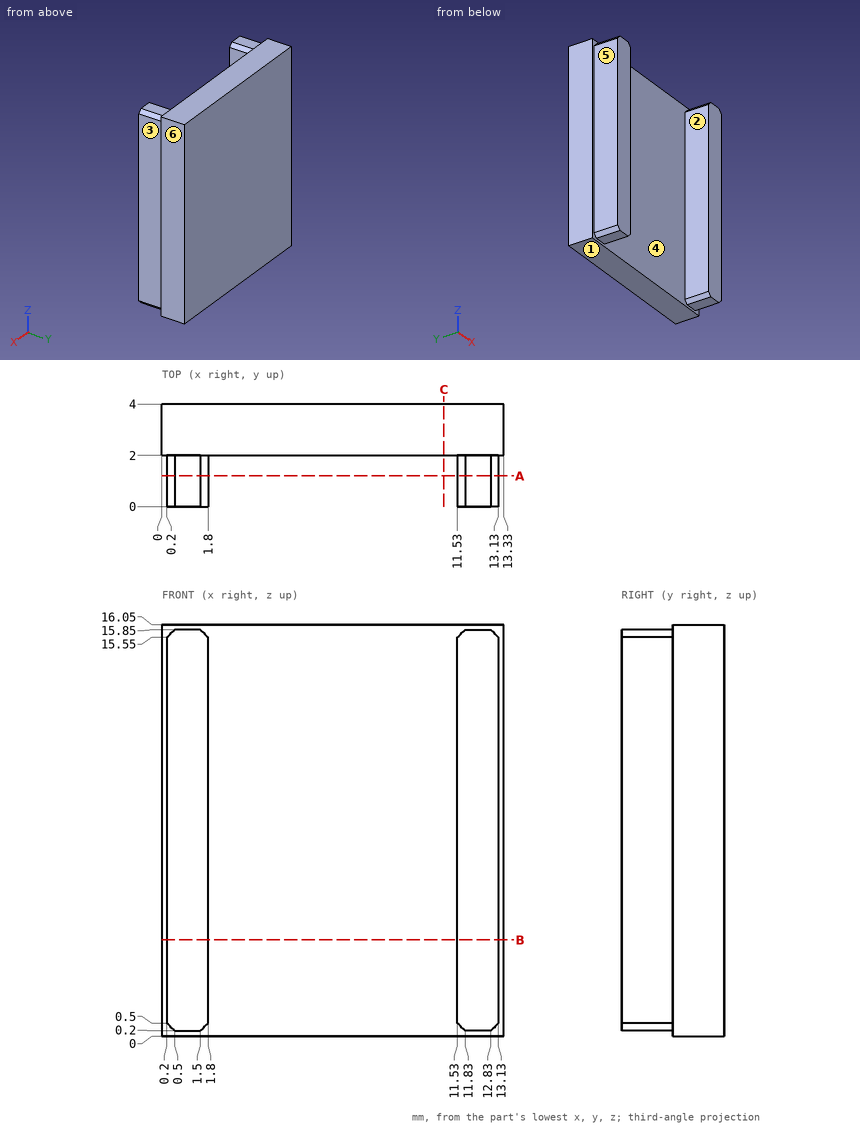
Can you work these out from the drawing? Everything is in mm from the part's minimum corner. A direction names the side the tool comes from. Coordinates: 2 decimals unless noted, no trailing zeros. Loops run counter-clockwise (first coordinate to the right, second up) from the corner with the lowest first, then second, coordinate; pieces in that order, holes last. Notation, with made-up numbers: (46.25, -31.75) - (72.25, -31.75) arc R20 cw to (72.25, -9.75) - close; hole circle Ø9 at (48.25, 11.25). An arc over 180 degrees is marked (long way). Use a Markdown table: item, result.
Item 1: Will these pins go through, and if not, where does the flat tip stop? pin 1 (1.1 mm diameter, centred on x = 12, y = 0.5, fed in from -Z); pin 2 (1.6 mm diameter, centred on y = 1, z = 11.5, fed in from -X).
Numbers:
| item | result |
|---|---|
| pin 1 | stops at z = 0.2 |
| pin 2 | stops at x = 0.2 |
Item 2: I want a section at C-C on x = 11. Please give me the cut outline in (y, z).
Numbers:
| item | result |
|---|---|
| outline | (2, 0) - (4, 0) - (4, 16.05) - (2, 16.05) - close |
Item 3: For the marked faces 1, 2 and 3, which set-ups out of +Z, -Z, +X, -X, +Y, -Y let a thin tool reach every point of the face, with its end or its side?
Numbers:
| item | result |
|---|---|
| face 1 | -Z, +X, -X, +Y, -Y |
| face 2 | +Z, -Z, -Y |
| face 3 | +Z, -Z, +X, -Y |
Item 4: We'd pull the mould along X, two halves only. Please class the marked faces 4, 5 and 6: released by +X, released by -X, zero draft, split by the parting line, or undercut.
Numbers:
| item | result |
|---|---|
| face 4 | undercut |
| face 5 | released by -X |
| face 6 | released by +X |
Item 5: If I drill on probe 1 along X at (y, z) = (1.7, 10.75); probe 2 along Y at (x, z) = (11, 13), over which ranges is the centre line in solid material (lowest first)? Write a range as from..to.
Numbers:
| item | result |
|---|---|
| probe 1 | x = 0.2..1.8, 11.53..13.13 |
| probe 2 | y = 2..4 |
Item 6: I want a section at A-A on y = 1.2. Please give me the cut outline in (x, z).
Numbers:
| item | result |
|---|---|
| outline | (0.2, 0.5) - (0.5, 0.2) - (1.5, 0.2) - (1.8, 0.5) - (1.8, 15.55) - (1.5, 15.85) - (0.5, 15.85) - (0.2, 15.55) - close; (11.53, 0.5) - (11.83, 0.2) - (12.83, 0.2) - (13.13, 0.5) - (13.13, 15.55) - (12.83, 15.85) - (11.83, 15.85) - (11.53, 15.55) - close |
Item 7: I want a section at B-B on z = 3.75. Please give me the cut outline in (x, y), and give its area (3 significant figures).
Numbers:
| item | result |
|---|---|
| outline | (0, 2) - (0.2, 2) - (0.2, 0) - (1.8, 0) - (1.8, 2) - (11.53, 2) - (11.53, 0) - (13.13, 0) - (13.13, 2) - (13.33, 2) - (13.33, 4) - (0, 4) - close |
| area | 33.1 mm2 |
